Autodesk Fusion 360 part; units mm, degrees
sketch "Sketch1" plane through (0, 0, 0) normal (0, 0, 1) x (1, 0, 0)
  line L0 (0, 0) -> (45.9912, 0)
  line L1 (45.9912, 0) -> (45.9912, 34.6951)
  line L2 (45.9912, 34.6951) -> (0, 34.6951)
  line L3 (0, 34.6951) -> (0, 0)
  circle A0 centre (22.9956, 17.3476) radius 7.8928
extrude "Extrude1" add sketch "Sketch1" against normal blind 24.87 contours L0 L1 L2 L3 | A0
extrude "Extrude2" add sketch "Sketch1" along normal blind 36.956 contours A0
fillet "Fillet1" radius 10.316 1 edges at (45.9912, 0, -12.435)
shell "Shell1" thickness 1.528 removed faces 1 at (18.3486, 16.3767, 36.956)
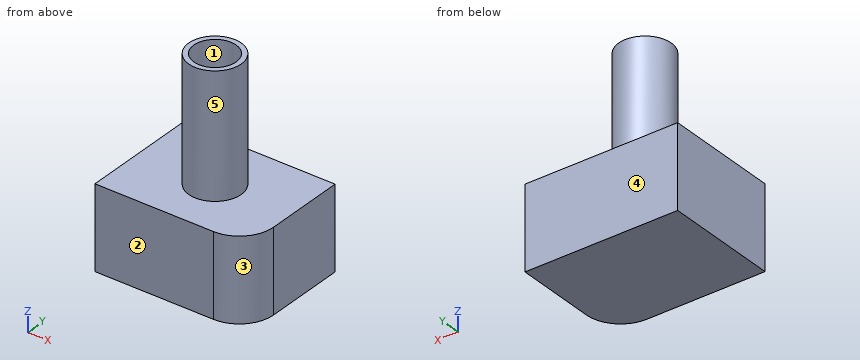
Part model, mm, in its own coordinate system. Face numbers are marked on the shaded views. A direction names the side the tool comes from. Round coordinates to 2 decimals unless told otherwise and drop trailing zeros. Write each loop counter-clockwise with the first axis right and the second up, starting at its lowest first coordinate (ties: lowest second). Pieces come first, ordered by that corner, then holes. Notation, with made-up numbers: M 22,2 L 48,2 A27 cw 48,29 Z; hole C 40.25,86.5 d2. An arc over 180 degrees is marked long. One line per question, with ' | ' between items.
(1) Two-plate mould, pull along X, no slides. Class the marked faces 1, 2 and 3: released by +X, released by -X, zero draft, split by the parting line, or undercut.
Answer key:
face 1: undercut | face 2: zero draft | face 3: released by +X
(2) 3-axis set-ups, long thin cutter, end or side, ignore diameter. For the marked faces 4 and 5: which of +Z, -Z, +X, -X, +Y, -Y reach the whole face in a straight line?
Answer key:
face 4: +Z, -Z, +X, -X, +Y | face 5: +Z
(3) Saw through at D-D on y = 19. Write the cut outline in (x, z).
Answer key:
outline: M 0,-24.87 L 45.99,-24.87 L 45.99,0 L 30.71,0 L 30.71,36.96 L 29.14,36.96 L 29.14,-1.53 L 44.46,-1.53 L 44.46,-23.34 L 1.53,-23.34 L 1.53,-1.53 L 16.85,-1.53 L 16.85,36.96 L 15.28,36.96 L 15.28,0 L 0,0 Z
(4) Saw through at C-C on y = 31.5. Write the cut outline in (x, z).
Answer key:
outline: M 0,-24.87 L 45.99,-24.87 L 45.99,0 L 0,0 Z; hole M 1.53,-23.34 L 44.46,-23.34 L 44.46,-1.53 L 1.53,-1.53 Z
(5) Pin check, flat tips, straight feed: pin 1 (3 mm diameter, centred on x = 25, z = 13, fed in from +Y); pin 2 (3 mm diameter, centred on x = 28, z = 7.5, fed in from -Y); pin 3 (8 mm diameter, centred on x = 13, z = 16.5, fed in from +Y). Stop position of each tip, or through.
Answer key:
pin 1: stops at y = 25.22 | pin 2: stops at y = 10.28 | pin 3: stops at y = 22.48
(6) Saw through at A-A on z = -7.5. Write the cut outline in (x, y).
Answer key:
outline: M 0,0 L 35.68,0 A10.32 ccw 45.99,10.32 L 45.99,34.7 L 0,34.7 Z; hole M 1.53,1.53 L 35.68,1.53 A8.79 ccw 44.46,10.32 L 44.46,33.17 L 1.53,33.17 Z
(7) Saw through at B-B on x = 14. Write the cut outline in (y, z).
Answer key:
outline: M 0,-24.87 L 34.7,-24.87 L 34.7,0 L 0,0 Z; hole M 1.53,-23.34 L 33.17,-23.34 L 33.17,-1.53 L 1.53,-1.53 Z
(8) Probe line 1 along Z through (x, y) = (13.5, 3); line 2 along X through (y, z) = (14.5, -17); line 3 along Z through (x, y) = (28, 11.5). List the from-to ranges inside material, lowest first.
Answer key:
line 1: z = -24.87 to -23.34, -1.53 to 0 | line 2: x = 0 to 1.53, 44.46 to 45.99 | line 3: z = -24.87 to -23.34, -1.53 to 36.96
